```python
from build123d import *

# Parameters (mm, degrees)
SKETCH1_W           = 100
SKETCH1_H           = 100
BOSS_EXTRUDE1_DEPTH = 30
BOSS_EXTRUDE2_DEPTH = 100
SKETCH4_R           = 35
BOSS_EXTRUDE3_DEPTH = 40


with BuildPart() as part:
    # Sketch1 → Boss-Extrude1 (new body)
    with BuildSketch(Plane.XY):
        with Locations((50, 50)):
            Rectangle(SKETCH1_W, SKETCH1_H)
    extrude(amount=BOSS_EXTRUDE1_DEPTH)

    # Sketch2 → Boss-Extrude2 (add)
    with BuildSketch(Plane(origin=(0, 0, 0), x_dir=(0, 0, -1), z_dir=(1, 0, 0))):
        Polygon((-30, 100), (-405.545697471, 266.651744151), (-459.843779827, 625.256045564), (-92.290312011, 856.669682909), (-92.290312011, 935.622570944), (-526.435767621, 651.422136489), (-459.843779827, 230.355875203), (-30, 0), align=None)
    extrude(amount=BOSS_EXTRUDE2_DEPTH)

    # Sketch4 → Boss-Extrude3 (add)
    with BuildSketch(Plane(origin=(0, 0, 92.290312011), x_dir=(-1, 0, 0), z_dir=(0, 0, -1))):
        with Locations((-50, 896.146126927)):
            Circle(SKETCH4_R)
    extrude(amount=BOSS_EXTRUDE3_DEPTH)


solid = part.part
```
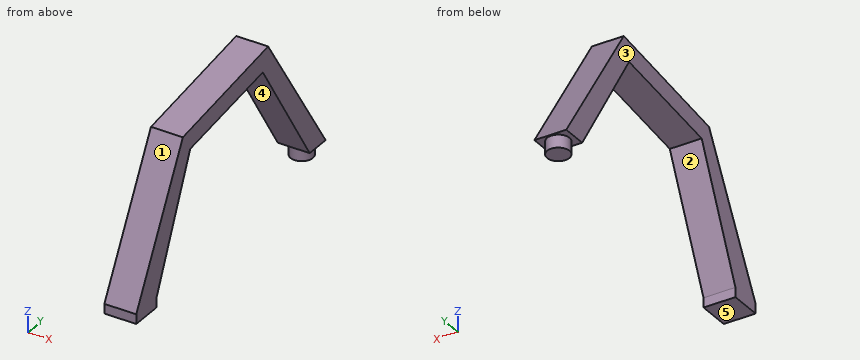
Work out the finished part from the listing and answer in its coordinate system (mm). Face numbers are marked on the shaded views. A direction names the side the tool comes from. Give positions to 0.01 mm unless a question says otherwise; leave off trailing zeros. Loops run counter-clockwise (first coordinate to the right, second up) from the corner with the lowest first, then second, coordinate; pieces in that order, holes last. Notation, with made-up numbers: (-5.5, 46) -> (44.5, 46) arc R25 ccw to (44.5, 78) -> close; hole circle Ø8 at (30.5, -8.75). An arc over 180 degrees is marked (long way). Use CSV: the item, a comma, the result in double quotes.
1. The part is cut by section A-A (z = 201). Write down the section's boundary in (x, y).
Found:
outline,"(0, 91.64) -> (100, 91.64) -> (100, 175.88) -> (0, 175.88) -> close; (0, 788.23) -> (100, 788.23) -> (100, 864.46) -> (0, 864.46) -> close"
2. Straight lines are drawn through the part: line 1 (Y direction, x = 82.5, z = 352); line 2 (Y direction, x = 5, z = 293); line 3 (Z direction, x = 76, y = 794). For each, find the intervals that lie inside material, in ascending order.
Found:
line 1,"172.56 to 242.89, 693.16 to 765.61"
line 2,"140.94 to 216.71, 730.3 to 804.23"
line 3,"191.83 to 308.63"
3. The mould has two halves that part along Y. Classify the marked faces 1, 2 and 3: +Y half, -Y half, draft (parallel to the pull), parting line (faces both ways), or undercut.
Found:
face 1,"-Y half"
face 2,"undercut"
face 3,"draft"
4. The part is cut by section B-B (x = 50). Write down the section's boundary in (y, z).
Found:
outline,"(0, 0) -> (100, 0) -> (100, 30) -> (266.65, 405.55) -> (625.26, 459.84) -> (856.67, 92.29) -> (861.15, 92.29) -> (861.15, 52.29) -> (931.15, 52.29) -> (931.15, 92.29) -> (935.62, 92.29) -> (651.42, 526.44) -> (230.36, 459.84) -> (0, 30) -> close"
5. Flat-ended cylindrical pins translate along their axes: pin 1 Ø12 at (x, y) = (67, 587) entering from -Z; pin 2 Ø3 at (x, y) = (55.5, 563.5) entering from +Z; pin 3 Ø1.5 at (x, z) = (36, 278.5) entering from +Y. Find the tip coordinate at first contact, or state that the pin passes through.
Found:
pin 1,"z = 453.14"
pin 2,"z = 512.77"
pin 3,"y = 814.22"
6. The part is cut by section D-D (y = 254.5). Write down the section's boundary in (x, z), then the cut area to 3 significant figures.
Found:
outline,"(0, 378.16) -> (100, 378.16) -> (100, 463.66) -> (0, 463.66) -> close"
area,"8,550 mm^2"
7. A tool of negligible diameter and unlimited length cuts with its end or side. For the marked faces 4 and 5, from which of +Z, -Z, +X, -X, +Y, -Y can it reach the whole face along a straight path? Write none if from no direction.
Found:
face 4,"-Z, +X, -X"
face 5,"-Z, +X, -X, +Y, -Y"
8. The part is cut by section C-C (z = 101.5). Write down the section's boundary in (x, y), then the cut area to 3 significant figures.
Found:
outline,"(0, 38.32) -> (100, 38.32) -> (100, 131.73) -> (0, 131.73) -> close; (0, 850.87) -> (100, 850.87) -> (100, 929.59) -> (0, 929.59) -> close"
area,"17,200 mm^2"
